Autodesk Inventor part; units mm, degrees
ref_plane "YZ Plane" through (0, 0, 0) normal (1, 0, 0) x (0, 1, 0)
ref_plane "XZ Plane" through (0, 0, 0) normal (0, 1, 0) x (-1, 0, 0)
ref_plane "XY Plane" through (0, 0, 0) normal (0, 0, 1) x (1, 0, 0)
sketch "Sketch1" plane through (0, 0, 0) normal (0, 0, 1) x (1, 0, 0)
  line L0 (0, -9.5) -> (0, 11.5)
  line L1 (-4, 7.5) -> (4, 7.5)
  line L2 (4, 7.5) -> (4, 2.1599)
  line L3 (4, 2.1599) -> (-4, 2.1599)
  line L4 (-4, 2.1599) -> (-4, 7.5)
  line L5 (-7, 0) -> (7, 0)
  line L6 (-4, 7.5) -> (-5, 4.34)
  line L7 (4, 7.5) -> (5, 4.34)
  line L8 (-4, 4.34) -> (4, 4.34)
  line L9 (-5, -6.5) -> (-5, 4.34)
  line L10 (5, 4.34) -> (5, -6.5)
  line L11 (5, -6.5) -> (-5, -6.5)
  line L12 (-4, 7.5) -> (4, 7.5)
  line L13 (4, 7.5) -> (4, 8.5)
  line L14 (4, 8.5) -> (-4, 8.5)
  line L15 (-4, 8.5) -> (-4, 7.5)
  point P0 (0, 7.5)
  point P1 (0, 0)
  dimension "d6" = 8
  dimension "d9" = 10.84
  dimension "d40" = 7.5
  dimension "d41" = 8.5
extrude "Plate1" add sketch "Sketch1" along normal blind 0.5
sketch "Sketch2" plane through (0, 0, 0.5) normal (0, 0, 1) x (1, 0, 0)
  circle A0 centre (0, 0) radius 2.5019
  line L0 (0, -9.5) -> (0, 11.5)
  point P0 (0, -3.9878)
  dimension "d12" = 5.0038
  dimension "d69" = 3.9878
extrude "Cut1" cut sketch "Sketch2" against normal blind 0.5
hole "Hole1" at (0, -3.9878, 0.5) direction (0, 0, -1) diameter 1.778 end through all
pattern_circular "Circular Pattern1" count 3 over 360 about axis through (0, 0, -10) along (0, 0, 1) of "Hole1"
sketch "Sketch3" plane through (0, 0, 0.5) normal (0, 0, 1) x (1, 0, 0)
  circle A0 centre (0, 0) radius 2.5019
  line L0 (-2.5, 5.334) -> (2.5, 5.334)
  line L1 (2.5, 5.334) -> (2.5, 4.572)
  line L2 (2.5, 4.572) -> (-2.5, 4.572)
  line L3 (-2.5, 4.572) -> (-2.5, 5.334)
  point P0 (0, 5.334)
  dimension "d25" = 5
  dimension "d26" = 0.762
  dimension "d27" = 5.334
cut "Cut2" [suppressed]
sketch "Sketch5" plane through (4, 8.9532, -0.2887) normal (0, 0.9063078, 0.4226183) x (-1, 0, 0)
  line L0 (8, 0) -> (0, 0)
  line L1 (0, 0) -> (0, -4.3629)
  line L2 (0, -4.3629) -> (8, -4.3629)
  line L3 (8, -4.3629) -> (8, 0)
edge flange "Flange2" height 5 angle 65 thickness 0.5 bend radius 0.5 thickness toward (0, 0.9063078, 0.4226183) relief tear relief width 0.5 relief depth 0.25 edges at (0, 8.5, 0) wall of the first edge with corners at (-4, 8.9532, -0.2887) (4, 8.9532, -0.2887) (4, 10.797, -4.2428) (-4, 10.797, -4.2428)
bend "Bend2"
corner "Corner2"
sketch "Sketch6" plane through (-4, 10.8363, -4.3673) normal (0, 0.9848078, 0.1736482) x (1, 0, 0)
  line L0 (8, 0) -> (0, 0)
  line L1 (0, 0) -> (0, -12.9342)
  line L2 (0, -12.9342) -> (8, -12.9342)
  line L3 (8, -12.9342) -> (8, 0)
edge flange "Flange3" height 13 angle -15 thickness 0.5 bend radius 0.5 thickness toward (0, 0.9848078, 0.1736482) relief tear relief width 0.5 relief depth 0.25 edges at (0, 11.2502, -4.0315) wall of the first edge with corners at (4, 10.8363, -4.3673) (-4, 10.8363, -4.3673) (-4, 13.0823, -17.105) (4, 13.0823, -17.105)
bend "Bend3"
corner "Corner3"
sketch "Sketch8" plane through (-4, 13.5747, -17.0182) normal (0, 0.9848078, 0.1736482) x (1, 0, 0)
  line L0 (0, -12.9342) -> (8, -12.9342)
  line L1 (8, -12.9342) -> (8, 0)
  line L2 (8, 0) -> (0, 0)
  line L3 (0, -12.9342) -> (0, 0)
  line L4 (2, 0) -> (6, 0)
  line L5 (6, 0) -> (6, -10.36)
  line L6 (6, -10.36) -> (2, -10.36)
  line L7 (2, -10.36) -> (2, 0)
  line L8 (4, 5.07) -> (4, -29.8212)
  line L9 (2, 0) -> (0, -7.32)
  line L10 (6, 0) -> (8, -7.32)
  line L11 (0, -7.32) -> (0, 0)
  line L12 (2, 0) -> (0, 0)
  line L13 (6, 0) -> (8, 0)
  line L14 (8, -7.32) -> (8, 0)
  point P0 (4, -19.1169)
  point P1 (4, 0)
  point P2 (4, 0)
  dimension "d63" = 4
  dimension "d64" = 7.32
  dimension "d65" = 12.9342
extrude "Cut3" cut sketch "Sketch8" against normal blind 0.5 contours L3 L2 L9 | L10 L2 L1
sketch "Sketch9" plane through (5, -6.5, 0) normal (1, 0, 0) x (0, 0, -1)
  line L0 (-0.5, 10.84) -> (-0.5, 0)
  line L1 (0, 0) -> (-0.5, 0)
  line L2 (0, 0) -> (0, 10.84)
  line L3 (0, 10.84) -> (-0.5, 10.84)
  line L4 (0.0774, 15.9063) -> (0.2887, 15.4532)
  arc A0 (0.0774, 15.9063) -> (-0.5, 15) centre (0.5, 15) ccw
  line L5 (0, 15) -> (-0.5, 15)
  arc A1 (0.2887, 15.4532) -> (0, 15) centre (0.5, 15) ccw
  line L6 (0, 14) -> (0, 15)
  line L7 (4.2805, 17.8287) -> (4.3673, 17.3363)
  arc A2 (4.2805, 17.8287) -> (4.0315, 17.7502) centre (4.4542, 16.8439) ccw
  line L8 (4.2428, 17.297) -> (4.0315, 17.7502)
  arc A3 (4.3673, 17.3363) -> (4.2428, 17.297) centre (4.4542, 16.8439) ccw
  line L9 (-0.5, 15) -> (15.0848, 17.748)
  line L10 (0.0774, 15.9063) -> (4.0315, 17.7502)
  point P0 (0, 6.5)
sketch "Sketch10" plane through (0, 0, 0.5) normal (0, 0, 1) x (1, 0, 0)
  circle A0 centre (0, 0) radius 2.5019
  line L0 (-2.54, 5.7658) -> (2.54, 5.7658)
  line L1 (2.54, 5.7658) -> (2.54, 4.4958)
  line L2 (2.54, 4.4958) -> (-2.54, 4.4958)
  line L3 (-2.54, 4.4958) -> (-2.54, 5.7658)
  point P0 (0, 5.7658)
  dimension "d70" = 1.27
  dimension "d71" = 5.08
  dimension "d72" = 4.4958
extrude "Cut4" cut sketch "Sketch10" against normal blind 0.5 contours L0 L1 L2 L3
equation "\"d13\" = Thickness"
equation "\"d20\" = Thickness"
equation "\"d28\" = Thickness"
equation "\"d66\" = Thickness"
equation "\"d73\" = Thickness"
equation "\"d42\" = BendReliefWidth"
equation "\"d43\" = BendReliefDepth"
equation "\"d44\" = MinimumRemnant"
equation "\"d45\" = BendRadius"
equation "\"d48\" = BendRadius"
equation "\"d49\" = CornerReliefSize"
equation "\"d50\" = GapSize"
equation "\"d51\" = JacobiRadiusSize"
equation "\"d52\" = BendReliefWidth"
equation "\"d53\" = BendReliefDepth"
equation "\"d54\" = MinimumRemnant"
equation "\"d55\" = BendRadius"
equation "\"d58\" = BendRadius"
equation "\"d59\" = CornerReliefSize"
equation "\"d60\" = GapSize"
equation "\"d61\" = JacobiRadiusSize"
equation "\"BendRadius\" = Thickness"
equation "\"BendReliefWidth\" = Thickness"
equation "\"BendReliefDepth\" = 0.5 * Thickness"
equation "\"CornerReliefSize\" = 4 * Thickness"
equation "\"MinimumRemnant\" = 2 * Thickness"
equation "\"TransitionRadius\" = BendRadius"
equation "\"JacobiRadiusSize\" = BendRadius"
equation "\"GapSize\" = Thickness"
equation "\"d10\" = BendRadius"
properties part number "ASAP_Top_Fixture_New(o)"
Geometry: final body of the model. Coordinates: model frame, mm. A direction names the side the tool comes from. Round coordinates to 2 decimals unless told otherwise and drop trailing zeros. Loops run counter-clockwise (first coordinate to the right, second up) from the corner with the lowest first, then second, coordinate; pieces in that order, holes last. Notation, with made-up numbers: (-28, 33.25) - (-22, 33.25) arc R28 cw to (-22, 52.25) - close; hole circle Ø10 at (36, 78). An arc over 180 degrees is marked (long way). Write each question's results on one line, items separated by ' | '. Start each with the question number.
1) Cut plane D-D on y = 5.5. Return loops of the section in (x, z).
2) Line query: probe 1 along Y at (x, z) = (0, 0.35); probe 2 along Z at (x, y) = (-3.25, 8.25); probe 3 along Y at (x, z) = (0, 0.2). Output: solid intervals per line, ascending. Write a range as [from, to].
3) Mould query, pull axis Y, two halves, no side actions, for faces 4 (the face through (-4.335, 2.11, 0.246)), 5 (the face through (0.056, 9.862, -2.238)), 6 (the face through (0, 3, 0)). Classes: released by +Y, released by -Y, zero draft, split by the parting line, or undercut.
4) Cut plane C-C on x = 2.25. Return loops of the section in (y, z), then the cut area to 3 significant figures.
5) Access query for faces 1 (the face through (-4, 11, -4)), 2 (the face through (4, 11, -4)), 3 (the face through (0.06, 10.34, -2.08)). Directions: +Z, -Z, +X, -X, +Y, -Y. A direction counts if a zero-diameter tool reaches every point of the face in a straight line with its end or side. Return the directions, or none.
6) Cut plane A-A on y = 0. Return loops of the section in (x, z).
7) First-contact query: P1, Ø1.6, axis at x = 3.45, y = 1.99, coming from the +Z side; P2, Ø4, axis at x = 0, y = 7, coming from the -Z side; P3, Ø3, axis at x = -1.5, y = 4.5, coming from the -Z side; P4, Ø0.6, axis at y = 5, z = 0.5, coming from the +X side. Flat tips, straight axial feed; report the tip coordinate or a pass-through.
8) Cut plane B-B on x = 0. Return loops of the section in (y, z) (3 decimals), then the cut area to 3 significant figures.
Verdict:
1) outline: (-4.63, 0) - (-2.54, 0) - (-2.54, 0.5) - (-4.63, 0.5) - close; (2.54, 0) - (4.63, 0) - (4.63, 0.5) - (2.54, 0.5) - close
2) probe 1: y = [-6.5, -4.88], [-3.1, -2.5], [2.5, 4.5], [5.77, 9.03] | probe 2: z = [0, 0.5] | probe 3: y = [-6.5, -4.88], [-3.1, -2.5], [2.5, 4.5], [5.77, 9.21]
3) face 4: undercut | face 5: released by -Y | face 6: zero draft
4) outline: (-6.5, 0) - (-1.09, 0) - (-1.09, 0.5) - (-6.5, 0.5) - close; (1.09, 0) - (4.5, 0) - (4.5, 0.5) - (1.09, 0.5) - close; (5.77, 0) - (8.5, 0) arc R0.5 cw to (8.95, -0.29) - (10.8, -4.24) arc R0.5 cw to (10.84, -4.37) - (12.92, -16.2) - (13.42, -16.12) - (11.33, -4.28) arc R1 ccw to (11.25, -4.03) - (9.41, -0.08) arc R1 ccw to (8.5, 0.5) - (5.77, 0.5) - close | area: 14.5 mm2
5) face 1: +Z, -Z, -X, +Y | face 2: +Z, -Z, +X, +Y | face 3: +Z, +X, -X, +Y
6) outline: (-5, 0) - (-2.5, 0) - (-2.5, 0.5) - (-5, 0.5) - close; (2.5, 0) - (5, 0) - (5, 0.5) - (2.5, 0.5) - close
7) P1: passes through | P2: stops at z = -0.39 | P3: stops at z = 0 | P4: stops at x = 4.89
8) outline: (-6.5, 0) - (-4.877, 0) - (-4.877, 0.5) - (-6.5, 0.5) - close; (-3.099, 0) - (-2.502, 0) - (-2.502, 0.5) - (-3.099, 0.5) - close; (2.502, 0) - (4.496, 0) - (4.496, 0.5) - (2.502, 0.5) - close; (5.766, 0) - (8.5, 0) arc R0.5 cw to (8.953, -0.289) - (10.797, -4.243) arc R0.5 cw to (10.836, -4.367) - (13.082, -17.105) - (13.575, -17.018) - (11.329, -4.281) arc R1 ccw to (11.25, -4.032) - (9.406, -0.077) arc R1 ccw to (8.5, 0.5) - (5.766, 0.5) - close | area: 12.6 mm2
